Source: CAD feature listing. Evaluate the final solid. Frame: model axes, mm. A direction names the side the tool comes from. Give positions to 0.01 mm unless a question says otherwise; leave off trailing zeros. Write each loop counter-clockwise with the first axis right and the second up, starting at its lowest first coordinate (ties: lowest second). Pieces come first, ordered by that corner, then holes.
```python
from build123d import *

# Parameters (mm, degrees)
F0_W     = 50
F0_H     = 66
F1_DEPTH = 50
F2_W     = 24
F2_H     = 15
F3_DEPTH = 100
F5_DEPTH = 100
F6_W     = 14
F6_H     = 16
F7_DEPTH = 100


with BuildPart() as f1:
    # F0 (on Top) → F1 (new body)
    with BuildSketch(Plane.XY):
        Rectangle(F0_W, F0_H)
    extrude(amount=-F1_DEPTH)

    # F2 (on face) → F3 (cut)
    with BuildSketch(Plane.XZ.offset(33)):
        with Locations((-0.730263, -7.5)):
            Rectangle(F2_W, F2_H)
    extrude(amount=-F3_DEPTH, mode=Mode.SUBTRACT)

    # F4 (on face) → F5 (cut)
    with BuildSketch(Plane.XZ.offset(33)):
        with BuildLine():
            ThreePointArc((6, -33), (-4.242641, -28.757359), (0, -39))
            ThreePointArc((0, -39), (4.242641, -37.242641), (6, -33))
        make_face()
    extrude(amount=-F5_DEPTH, mode=Mode.SUBTRACT)

    # F6 (on face) → F7 (cut)
    with BuildSketch(Plane.XY.offset(-15)):
        with Locations((-0.993422, 15)):
            Rectangle(F6_W, F6_H)
        with Locations((-0.993422, -15)):
            Rectangle(F6_W, F6_H)
    extrude(amount=-F7_DEPTH, mode=Mode.SUBTRACT)


solid = f1.part
```
1. Section query A-A (z = -12). Return loops of the section in (x, y), plus the area to 3 significant figures.
2. Section query C-C (z = -21). Return loops of the section in (x, y).
3. Section query B-B (y = -20). Return loops of the section in (x, z), plus the area to 3 significant figures.
4. Access query for faces 1 (the flat face through (-12.73, 0, -8)), 2 (the flat face through (0, 33, -25)), 3 (the flat face through (-4, -23, -28)). Directions: +Z, -Z, +X, -X, +Y, -Y. A direction counts if a zero-diameter tool reaches every point of the face in a straight line with its end or side. Return the directions, or none.
5. Line query: probe 1 along Y at (x, z) = (-6.5, -41); probe 2 along Z at (x, y) = (0, -1.75); probe 3 along X at (y, z) = (14.5, -19.5). Output: solid intervals per line, ascending.
6. Pull-direction query (X, two-part tool) for faces 4 (the flat face through (6.007, -15, -32)), 5 (the flat face through (0, 0, -50)), 6 (the flat face through (-25, 0, -25)), 7 (the flat face through (25, 0, -25)); classes: pulls with the +X half, pulls with the -X half, needs draft (parallel to the pull), parting line crosses it, or undercut.
7. Pin query (flat end, axial travel): P1, Ø7, axis at x = 0, z = -33, coming from the +Y side. Return the tip coordinate at first contact, or that it passes through.
The answers:
1. outline: (-25, -33) - (-12.73, -33) - (-12.73, 33) - (-25, 33) - close; (11.27, -33) - (25, -33) - (25, 33) - (11.27, 33) - close
1. area: 1,720 mm2
2. outline: (-25, -33) - (25, -33) - (25, 33) - (-25, 33) - close; hole (-7.99, -23) - (6.01, -23) - (6.01, -7) - (-7.99, -7) - close; hole (-7.99, 7) - (6.01, 7) - (6.01, 23) - (-7.99, 23) - close
3. outline: (-25, -50) - (-7.99, -50) - (-7.99, -15) - (-12.73, -15) - (-12.73, 0) - (-25, 0) - close; (6.01, -50) - (25, -50) - (25, 0) - (11.27, 0) - (11.27, -15) - (6.01, -15) - close
3. area: 1,650 mm2
4. face 1: +Z, +Y, -Y
4. face 2: +Z, -Z, +X, -X, +Y
4. face 3: +Z, -Z
5. probe 1: y = -33 to -23, -7 to 7, 23 to 33
5. probe 2: z = -50 to -39, -27 to -15
5. probe 3: x = -25 to -7.99, 6.01 to 25
6. face 4: undercut
6. face 5: needs draft
6. face 6: pulls with the -X half
6. face 7: pulls with the +X half
7. P1: passes through
